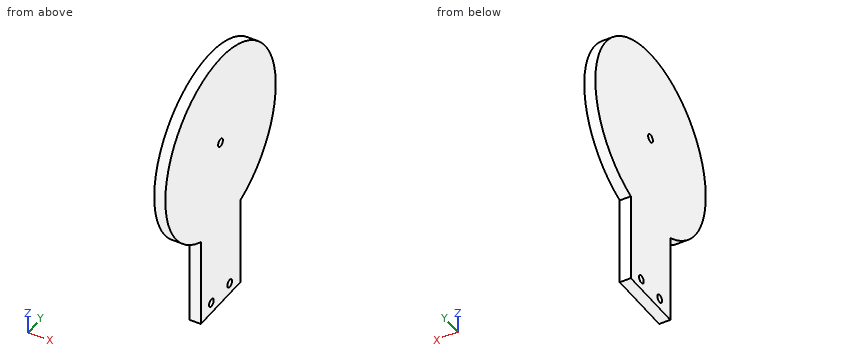
from build123d import *

# Parameters (mm, degrees)
EXTRUDE_1_DEPTH     = 2.5
SKETCH_2_R          = 0.9
CUT_EXTRUDE_1_DEPTH = 3.5


with BuildPart() as part:
    # 스케치1 → 보스-돌출1 (new body)
    with BuildSketch(Plane(origin=(-9, 0, 0), x_dir=(0, -1, 0), z_dir=(-1, 0, 0))):
        with BuildLine():
            Line((-21, -18.122865071), (-21, 2.262089683))
            ThreePointArc((-21, 2.262089683), (-13.5, 42.877134929), (-6, 2.262089683))
            Line((-6, 2.262089683), (-6, -18.122865071))
            Line((-6, -18.122865071), (-21, -18.122865071))
        make_face()
    extrude(amount=-EXTRUDE_1_DEPTH)

    # 스케치2 → 컷-돌출1 (cut, through all)
    with BuildSketch(Plane(origin=(-6.5, 0, 0), x_dir=(0, 0, -1), z_dir=(1, 0, 0))):
        with Locations((15.622865071, 10)):
            Circle(SKETCH_2_R)
        with Locations((15.622865071, 17)):
            Circle(SKETCH_2_R)
        with Locations((-21.877134929, 13.5)):
            Circle(SKETCH_2_R)
    extrude(amount=-CUT_EXTRUDE_1_DEPTH, mode=Mode.SUBTRACT)


solid = part.part
Geometry: final body of the model. Coordinates: model frame, mm. Give positions to 0.01 mm unless a question says otherwise; leave off trailing zeros. Order: outer loops, then holes, each group sorted by start corner. A loop starts at its lowest first (then second) coordinate and runs counter-clockwise, first axis right, second up. Notation, with made-up numbers: (-15, 55) -> (40, 55) arc R36 ccw to (40, 91) -> close; hole circle Ø2 at (31.25, 26). An arc over 180 degrees is marked (long way). Write each question's results on one line, items separated by ' | '.
1) Cut plane B-B (x = -8.3). Output: boundary loops of the cut face in (y, z), and give its area (3 significant figures).
Geometry says:
outline: (6, -18.12) -> (21, -18.12) -> (21, 2.26) arc R21 ccw (long way) to (6, 2.26) -> close; hole circle Ø1.8 at (10, -15.62); hole circle Ø1.8 at (13.5, 21.88); hole circle Ø1.8 at (17, -15.62) | area: 1,670 mm²
2) Cut plane C-C (z = 9). Output: boundary loops of the cut face in (x, y).
Geometry says:
outline: (-9, -3.09) -> (-6.5, -3.09) -> (-6.5, 30.09) -> (-9, 30.09) -> close
3) Cut plane A-A (y = 17). Output: boundary loops of the cut face in (x, z), and give its area (3 significant figures).
Geometry says:
outline: (-9, -18.12) -> (-6.5, -18.12) -> (-6.5, -16.52) -> (-9, -16.52) -> close; (-9, -14.72) -> (-6.5, -14.72) -> (-6.5, 42.58) -> (-9, 42.58) -> close | area: 147 mm²
4) Line query: line 1 along Z through (x, y) = (-7.15, 13); line 2 along Z through (x, y) = (-8.55, -4); line 3 along Z through (x, y) = (-8.45, 8.5). Output: solid intervals per line, ascending.
Geometry says:
line 1: z = -18.12 to 21.13, 22.63 to 42.87 | line 2: z = 10.27 to 33.49 | line 3: z = -18.12 to 42.27
5) Cut plane D-D (y = 24.5). Output: boundary loops of the cut face in (x, z).
Geometry says:
outline: (-9, 3.99) -> (-6.5, 3.99) -> (-6.5, 39.77) -> (-9, 39.77) -> close
6) First-contact query: pin 1 Ø3 at (y, z) = (13.5, 21.88) entering from +X; pin 2 Ø1 at (x, z) = (-8, -6) entering from +Y; pin 3 Ø1.1 at (y, z) = (17, -15.62) entering from -X. Flat tips, straight axial feed; report the tip coordinate or a pass-through.
Geometry says:
pin 1: stops at x = -6.5 | pin 2: stops at y = 21 | pin 3: passes through
